Could you check a few things on this drawing? It's one solid part, dimensions in mm from its lowest x, y, z. A direction names the side the tool comes from. Give positions to 0.01 mm unless a question says otherwise; leave off trailing zeros. Loops run counter-clockwise (first coordinate to the right, second up) from the corner with the lowest first, then second, coordinate; pieces in that order, holes last. Notation, with made-up numbers: (61, -3.5) - (113, -3.5) arc R23 cw to (113, 6.5) - close; hole circle Ø4 at (6, 79.5). An arc over 180 degrees is marked (long way). Answer as a JSON object with one key per item and string values.
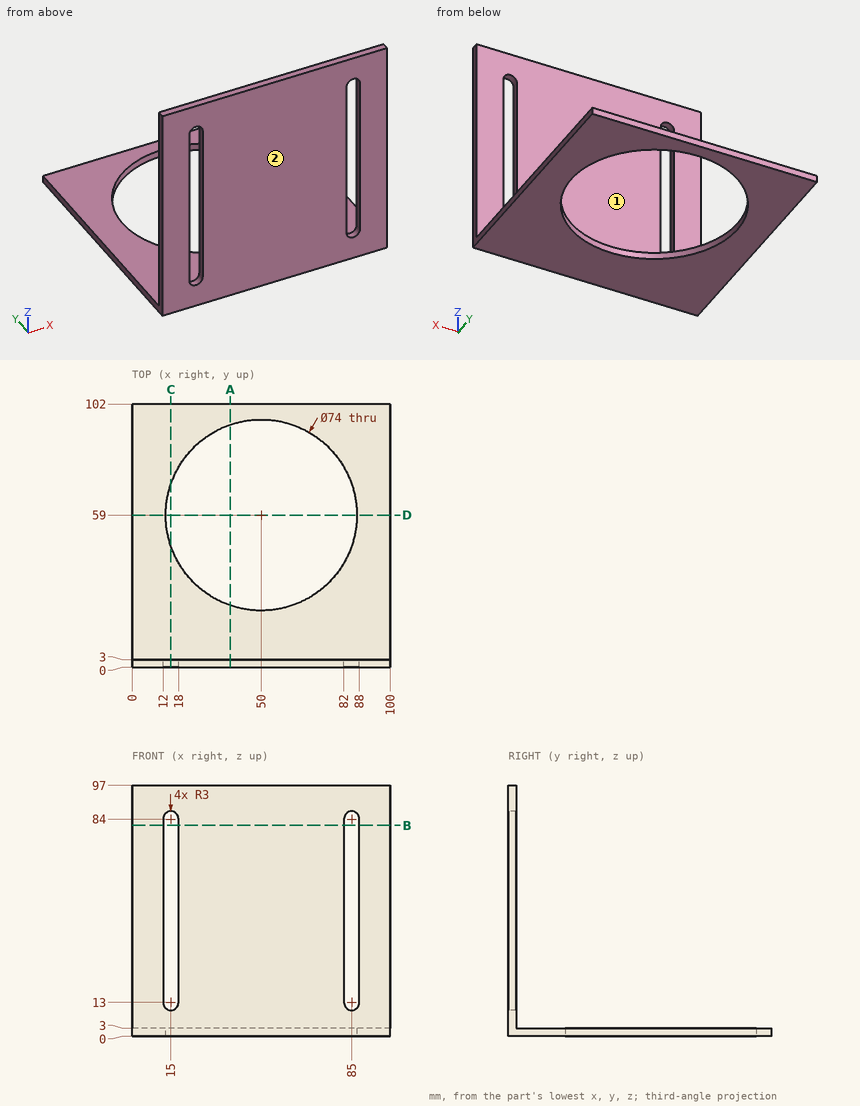
1) Imagine slicing it at B-B on z = 81.5. Write out the boundary of the cut face in (x, y).
Check sheet entries:
{"outline": "(0, 0) - (12, 0) - (12, 3) - (0, 3) - close; (18, 0) - (82, 0) - (82, 3) - (18, 3) - close; (88, 0) - (100, 0) - (100, 3) - (88, 3) - close"}
2) Imagine slicing it at A-A on x = 38. Write out the boundary of the cut face in (y, z).
Check sheet entries:
{"outline": "(0, 0) - (24, 0) - (24, 3) - (3, 3) - (3, 97) - (0, 97) - close; (94, 0) - (102, 0) - (102, 3) - (94, 3) - close"}
3) I need wall thicknesses on L1, parallel to Y at x = 50, z = 1; L2, parallel to Y at x = 60, z = 36. Which ranges of each line are inside material? Lowest first, please.
Check sheet entries:
{"L1": "0 to 22, 96 to 102", "L2": "0 to 3"}
4) Imagine slicing it at D-D on y = 59. Write out the boundary of the cut face in (x, z).
Check sheet entries:
{"outline": "(0, 0) - (13, 0) - (13, 3) - (0, 3) - close; (87, 0) - (100, 0) - (100, 3) - (87, 3) - close"}
5) Which directions (+Z, -Z, +X, -X, +Y, -Y) give clear straight access to the entire face, cutting with the end or side of a thin tool? Please do the marked faces 1 and 2.
Check sheet entries:
{"face 1": "+Z, +X, -X, +Y", "face 2": "+Z, -Z, +X, -X, -Y"}
6) I'm going to push a flat-ended pin straight in: P1, Ø1, axis at x = 39, z = 31.5, coming from the +Y side. Where does the tip first touch, or does it pass through?
Check sheet entries:
{"P1": "y = 3"}
7) Imagine slicing it at C-C on x = 15. Write out the boundary of the cut face in (y, z).
Check sheet entries:
{"outline": "(0, 0) - (47, 0) - (47, 3) - (3, 3) - (3, 10) - (0, 10) - close; (0, 87) - (3, 87) - (3, 97) - (0, 97) - close; (71, 0) - (102, 0) - (102, 3) - (71, 3) - close"}
